Autodesk Inventor part; units mm, degrees
ref_plane "YZ Plane" through (0, 0, 0) normal (1, 0, 0) x (0, 1, 0)
ref_plane "XZ Plane" through (0, 0, 0) normal (0, 1, 0) x (-1, 0, 0)
ref_plane "XY Plane" through (0, 0, 0) normal (0, 0, 1) x (1, 0, 0)
sketch "Sketch1" plane through (0, 0, 0) normal (0, 1, 0) x (-1, 0, 0)
  line L0 (0, 0) -> (230, 0)
  line L1 (230, 0) -> (230, -130)
  line L2 (230, -130) -> (0, -130)
  line L3 (0, -130) -> (0, 0)
  dimension "d0" = 130
  dimension "d1" = 230
extrude "Extrusion1" add sketch "Sketch1" along normal blind 5
sketch "Sketch2" plane through (0, 5, 0) normal (0, 1, 0) x (1, 0, 0)
  line L0 (-230, 130) -> (-230, 0)
  line L1 (0, 0) -> (0, 130)
  line L2 (-230, 0) -> (0, 0)
  line L3 (0, 0) -> (0, 130)
  line L4 (0, 130) -> (-230, 130)
  line L5 (-230, 130) -> (-230, 0)
  line L6 (-225, 5) -> (-5, 5)
  line L7 (-5, 5) -> (-5, 125)
  line L8 (-5, 125) -> (-225, 125)
  line L9 (-225, 125) -> (-225, 5)
  dimension "d4" = 5
  dimension "d6" = 5
  dimension "d7" = 5
  dimension "d8" = 5
extrude "Extrusion2" add sketch "Sketch2" along normal blind 70
sketch "Sketch3" plane through (0, 5, 0) normal (0, 1, 0) x (1, 0, 0)
  line L0 (-225, 5) -> (-5, 5)
  line L1 (-5, 125) -> (-225, 125)
  line L2 (-65, 5) -> (-70, 5)
  line L3 (-70, 5) -> (-70, 125)
  line L4 (-70, 125) -> (-65, 125)
  line L5 (-65, 125) -> (-65, 5)
  line L6 (-5, 125) -> (-5, 5)
  point P0 (0, 0)
  dimension "d11" = 5
  dimension "d12" = 60
extrude "Extrusion3" add sketch "Sketch3" along normal up to surface (70 mm away) contours L3 L1 L5 L0
sketch "Sketch4" plane through (-65, 5, -5) normal (1, 0, 0) x (0, 0, -1)
  circle A0 centre (60, 52.5) radius 7.5
  line L0 (120, 70) -> (0, 70)
  point P0 (-5, -5)
  point P1 (60, 70)
  point P2 (60, 70)
  point P3 (60, 70)
  dimension "d15" = 15
  dimension "d16" = 17.5
extrude "Extrusion4" cut sketch "Sketch4" against normal up to surface (5 mm away)
sketch "Sketch6" plane through (-225, 5, -125) normal (0, 0, 1) x (1, 0, 0)
  line L0 (155, 0) -> (0, 0)
  line L1 (0, 0) -> (155, 0)
  line L2 (155, 0) -> (0, 8.1232)
  line L3 (0, 0) -> (0, 70)
  line L4 (0, 8.1232) -> (0, 0)
  line L5 (160, 0) -> (220, 5.2493)
  line L6 (220, 0) -> (220, 70)
  line L7 (220, 5.2493) -> (220, 0)
  line L8 (220, 0) -> (160, 0)
  point P0 (225, -5)
  dimension "d38" = 5
  dimension "d39" = 3
extrude "Extrusion5" add sketch "Sketch6" along normal up to surface (120 mm away)
sketch "Sketch7" plane through (0, 75, 0) normal (0, 1, 0) x (1, 0, 0)
  line L0 (-225, 125) -> (-70, 125)
  line L1 (-70, 5) -> (-225, 5)
  line L2 (-70, 125) -> (-73, 125)
  line L3 (-73, 125) -> (-73, 5)
  line L4 (-73, 5) -> (-70, 5)
  line L5 (-70, 5) -> (-70, 125)
  line L6 (-65, 125) -> (-65, 5)
  line L7 (-65, 125) -> (-62, 125)
  line L8 (-62, 125) -> (-62, 5)
  line L9 (-62, 5) -> (-65, 5)
  line L10 (-65, 5) -> (-65, 125)
  point P0 (0, 0)
  point P1 (-71.5, 5)
  point P2 (-63.5, 5)
  dimension "d42" = 3
  dimension "d43" = 3
extrude "Extrusion6" cut sketch "Sketch7" against normal through all
sketch "Sketch8" plane through (0, 0, 0) normal (0, -1, 0) x (1, 0, 0)
  line L0 (-230, -130) -> (0, -130)
  line L1 (-230, 0) -> (-230, -130)
  line L2 (-230, -130) -> (-230, 0)
  line L3 (-230, -65) -> (0, -65)
  line L4 (0, -130) -> (0, 0)
  line L5 (-115, -130) -> (-115, 0)
  point P0 (-210, -115)
  point P1 (-210, -15)
  point P2 (-20, -115)
  point P3 (-20, -15)
  dimension "d46" = 15
  dimension "d47" = 20
hole "Hole2" at (-210, 0, -115) at (-210, 0, -15) at (-20, 0, -15) at (-20, 0, -115) direction (0, 1, 0) diameter 4 depth 7.5
sketch "Sketch9" plane through (-230, 0, 0) normal (0, 0, 1) x (1, 0, 0)
  line L0 (20, 65) -> (233.5105, 65)
  line L1 (20, 45) -> (233.5105, 45)
  line L2 (234.6135, 25) -> (20, 25)
  line L3 (0, 75) -> (230, 75)
  line L4 (0, 0) -> (0, 75)
  point P0 (230, 0)
  point P1 (30, 45)
  point P2 (40, 65)
  point P3 (50, 45)
  point P4 (40, 25)
  point P5 (60, 65)
  point P6 (70, 45)
  point P7 (60, 25)
  point P8 (80, 65)
  point P9 (90, 45)
  point P10 (80, 25)
  point P11 (100, 65)
  point P12 (110, 45)
  point P13 (100, 25)
  point P14 (120, 65)
  point P15 (130, 45)
  point P16 (120, 25)
  point P17 (140, 65)
  point P18 (150, 45)
  point P19 (140, 25)
  point P20 (170, 45)
  point P21 (180, 65)
  point P22 (190, 45)
  point P23 (180, 25)
  point P24 (200, 65)
  point P25 (210, 45)
  point P26 (200, 25)
  dimension "d55" = 20
  dimension "d56" = 20
  dimension "d57" = 10
  dimension "d58" = 20
  dimension "d59" = 10
  dimension "d62" = 20
hole "Hole3" at (-210, 65, 0) at (-200, 45, 0) at (-210, 25, 0) at (-190, 65, 0) at (-180, 45, 0) at (-190, 25, 0) at (-170, 65, 0) at (-160, 45, 0) at (-170, 25, 0) at (-150, 65, 0) at (-140, 45, 0) at (-150, 25, 0) at (-130, 65, 0) at (-120, 45, 0) at (-130, 25, 0) at (-110, 65, 0) at (-100, 45, 0) at (-110, 25, 0) at (-90, 65, 0) at (-80, 45, 0) at (-90, 25, 0) at (-50, 65, 0) at (-40, 45, 0) at (-50, 25, 0) at (-30, 65, 0) at (-20, 45, 0) at (-30, 25, 0) at (-60, 45, 0) direction (0, 0, -1) diameter 4 end through all
equation "\"d4\" = d8"
equation "\"d6\" = d7"
equation "\"d7\" = d8"
equation "\"d43\" = d42"
properties part number "bottomA"
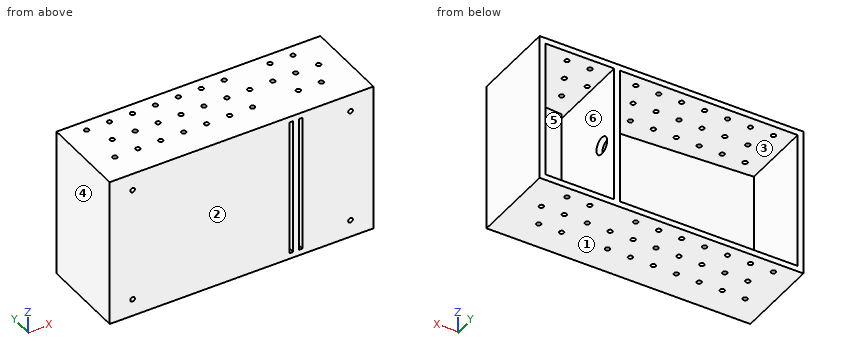
Read the model definition and answer for the solid it produces. Units are mm, in the model's axes. Face numbers are marked on the shaded views. A direction names the side the tool comes from. Coordinates: 2 decimals unless noted, no trailing zeros. Loops run counter-clockwise (first coordinate to the right, second up) from the corner with the lowest first, then second, coordinate; pieces in that order, holes last. Notation, with made-up numbers: (11, 45) -> (32, 45) arc R27 cw to (32, 81) -> close; hole circle Ø5 at (85, 8). An arc over 180 degrees is marked (long way). Answer in a Markdown table with one row per item.
Item 1: A cutting plane is placed at A-A on y = 33.5. Determine the outline of the cut face in (x, z), plus the area to 3 significant figures.
Returned:
| item | result |
|---|---|
| outline | (-230, -130) -> (0, -130) -> (0, 0) -> (-230, 0) -> close; hole (-225, -125) -> (-70, -125) -> (-70, -5) -> (-225, -5) -> close; hole (-65, -125) -> (-5, -125) -> (-5, -5) -> (-65, -5) -> close |
| area | 4,100 mm^2 |
Item 2: Straight lines are drawn through the part: line 1 along Y through (x, z) = (-110, -2.85); line 2 along X through (y, z) = (40.5, -33); line 3 along X through (y, z) = (4, -15). For each, find the intervals that lie inside material, in ascending order. Write a range as [from, to].
Returned:
| item | result |
|---|---|
| line 1 | y = [0, 23], [27, 63], [67, 75] |
| line 2 | x = [-230, -225], [-70, -65], [-5, 0] |
| line 3 | x = [-230, -212], [-208, -73], [-70, -65], [-62, -22], [-18, 0] |
Item 3: For a pull along Z with two mould halves and no side action, classify the marked faces 1, 2 and 3 as released by +Z, released by -Z, zero draft, split by the parting line, or undercut.
Returned:
| item | result |
|---|---|
| face 1 | released by -Z |
| face 2 | zero draft |
| face 3 | undercut |
Item 4: A cutting plane is placed at B-B on z = -107. Determine the outline of the cut face in (x, y), plus the area to 3 significant figures.
Returned:
| item | result |
|---|---|
| outline | (-230, 0) -> (-73, 0) -> (-73, 5.16) -> (-225, 13.12) -> (-225, 75) -> (-230, 75) -> close; (-70, 0) -> (-65, 0) -> (-65, 75) -> (-70, 75) -> close; (-62, 0) -> (0, 0) -> (0, 75) -> (-5, 75) -> (-5, 10.25) -> (-62, 5.26) -> close |
| area | 2,960 mm^2 |
Item 5: A cutting plane is placed at C-C on y = 55. Determine the outline of the cut face in (x, z), plus the area to 3 significant figures.
Returned:
| item | result |
|---|---|
| outline | (-230, -130) -> (0, -130) -> (0, 0) -> (-230, 0) -> close; hole (-225, -125) -> (-70, -125) -> (-70, -72.07) -> (-65, -72.07) -> (-65, -125) -> (-5, -125) -> (-5, -5) -> (-65, -5) -> (-65, -57.93) -> (-70, -57.93) -> (-70, -5) -> (-225, -5) -> close |
| area | 4,030 mm^2 |
Item 6: Each of these flat-tipped pins is pushed along its axis until it touches: P1, Ø2.5, axis at x = -180, y = 45, coming from the +Z side; P2, Ø10, axis at x = -52.5, z = -94.5, coming from the +Y side; P3, Ø3, axis at x = -62, z = -50.5, coming from the +Y side. Where does it stop, or does it pass through?
Returned:
| item | result |
|---|---|
| P1 | passes through |
| P2 | stops at y = 6.53 |
| P3 | stops at y = 5.39 |
Item 7: For the marked faces 4, 5 and 6, determine the directions among +Z, -Z, +X, -X, +Y, -Y from which every point of the face is accessible in a straight line to the end or side of a thin tool.
Returned:
| item | result |
|---|---|
| face 4 | +Z, -Z, -X, +Y, -Y |
| face 5 | +Y |
| face 6 | +Y, -Y |
